Design review of the part built by this model. Coordinates are the model's own, in mm. A direction names the side the tool comes from. Coordinates: 2 decimals unless noted, no trailing zeros. Order: outer loops, then holes, each group sorted by start corner. A loop starts at its lowest first (then second) coordinate and runs counter-clockwise, first axis right, second up.
from build123d import *

# Parameters (mm, degrees)
ESQUISSE1_R             = 1.65
BOSS_EXTRU_1_DEPTH      = 9
ESQUISSE2_R             = 0.75
ENL_V_MAT_EXTRU_1_DEPTH = 14.568806138


with BuildPart() as part:
    # Esquisse1 → Boss.-Extru.1 (new, symmetric)
    with BuildSketch(Plane.XY):
        with BuildLine():
            Line((0, -4.15), (0, -5.85))
            Line((0, -5.85), (4.15, -5.85))
            Line((4.15, -5.85), (4.15, 4.15))
            Line((4.15, 4.15), (0, 4.15))
            ThreePointArc((0, 4.15), (-4.15, 0), (0, -4.15))
        make_face()
        Circle(ESQUISSE1_R, mode=Mode.SUBTRACT)
    extrude(amount=BOSS_EXTRU_1_DEPTH, both=True)

    # Esquisse2 → Enlèv. mat.-Extru.1 (cut, through all)
    with BuildSketch(Plane(origin=(4.15, 0, 0), x_dir=(0, 0, -1), z_dir=(1, 0, 0))):
        with Locations((-6.35, -3.35)):
            Circle(ESQUISSE2_R)
        with Locations((6.35, -3.35)):
            Circle(ESQUISSE2_R)
    extrude(amount=-ENL_V_MAT_EXTRU_1_DEPTH, mode=Mode.SUBTRACT)


solid = part.part
1. Add section B-B (z = -6.35). Give the boundary of the cut face in (x, y).
2. Add section D-D (x = -1). Give the boundary of the cut face in (y, z).
3. Mouldability with a two-part tool opening along X and no side actions: class faces 3 (the flat face through (2, 4.15, 0)), 4 (the cylindrical face through (-1.216, 1.115, -0.126)), 5 (the flat face through (4.15, -1, 0)) as pulls with the +X half, pulls with the -X half, needs draft (parallel to the pull), parting line crosses it, or undercut.
4. Add section A-A (y = 0). Give the boundary of the cut face in (x, z), and give its area (3 significant figures).
5. Insertion check: pin 1 (1.5 mm diameter, centred on y = -1.5, z = 1, fed in from -X); pin 2 (2 mm diameter, centred on y = -3.35, z = -6.35, fed in from +X); pin 3 (0.8 mm diameter, centred on y = -5.5, z = 4.5, fed in from -X). Each pin has a flat end and moves straight along its axis. Give the tip position at first contact, or say it passes through.
6. Add section C-C (x = 3.75). Give the boundary of the cut face in (y, z).
7. For faces 1 (the cylindrical face through (1.3, -2.6, 6.4)), 2 (the flat face through (0, -5, 0)), list the 3-axis set-ups (+Z, -Z, +X, -X, +Y, -Y) from which the entire face can be reached by the end or side of a thin tool; tool diameter is ignored.
8. To check wall thickness, follow line 1 (Z direction, x = 1.75, y = -3.35); line 2 (Y direction, x = 0.25, z = -6.35); line 3 (X direction, y = -4.5, z = -5.5). State the ranges of each line that lie inside material, in increasing order.
Solution:
1. outline: (-3.23, -2.6) - (4.15, -2.6) - (4.15, 4.15) - (0, 4.15) arc R4.15 ccw to start; (-0.64, -4.1) arc R4.15 ccw to (0, -4.15) - (0, -5.85) - (4.15, -5.85) - (4.15, -4.1) - close; hole circle Ø3.3 at (0, 0)
2. outline: (-4.03, -9) - (-1.31, -9) - (-1.31, 9) - (-4.03, 9) - (-4.03, 6.67) arc R0.75 cw (long way) to (-4.03, 6.03) - (-4.03, -6.03) arc R0.75 cw (long way) to (-4.03, -6.67) - close; (1.31, -9) - (4.03, -9) - (4.03, 9) - (1.31, 9) - close
3. face 3: needs draft
3. face 4: undercut
3. face 5: pulls with the +X half
4. outline: (-4.15, -9) - (-1.65, -9) - (-1.65, 9) - (-4.15, 9) - close; (1.65, -9) - (4.15, -9) - (4.15, 9) - (1.65, 9) - close
4. area: 90.0 mm2
5. pin 1: stops at x = -4.08
5. pin 2: stops at x = 4.15
5. pin 3: stops at x = 0
6. outline: (-5.85, -9) - (4.15, -9) - (4.15, 9) - (-5.85, 9) - close; hole circle Ø1.5 at (-3.35, -6.35); hole circle Ø1.5 at (-3.35, 6.35)
7. face 1: +X, -X
7. face 2: +Z, -Z, -X, -Y
8. line 1: z = -9 to -7.1, -5.6 to 5.6, 7.1 to 9
8. line 2: y = -5.85 to -4.1, -2.6 to -1.63, 1.63 to 4.15
8. line 3: x = 0 to 4.15
